Answer from the drawing. Dimensions are ordinates in mm from the lowest x, y and z of the part. Coordinates: 2 decimals unless noted, no trailing zeros. Order: outer loops, then holes, each group sorted by start corner. A loop starts at its lowest first (then second) coordinate and runs counter-clockwise, first axis right, second up. Notation, with made-up numbers: (57, -6) -> (116, -6) arc R27 cw to (116, 23) -> close; hole circle Ø10 at (85.5, -17.5). An arc over 180 degrees is marked (long way). Answer as a JSON object with one key per item and string values. Group by question number.
1) Consider L1, parallel to Z at x = 4, y = 1.2; L2, parallel to Z at x = 26, y = 1; L3, parallel to X at y = 0.4, z = 37. Determine where each line is inside the solid, lowest interval first.
2) Section C-C on z = 67 is taken. Determine the outline of the cut face in (x, y).
3) Section D-D on z = 35.5 is taken. Determine the outline of the cut face in (x, y), and give its area (3 significant figures).
4) Section A-A on y = 1.45 is taken. Determine the outline of the cut face in (x, z).
5) Section B-B on x = 4 is taken. Determine the outline of the cut face in (y, z), and give its area (3 significant figures).
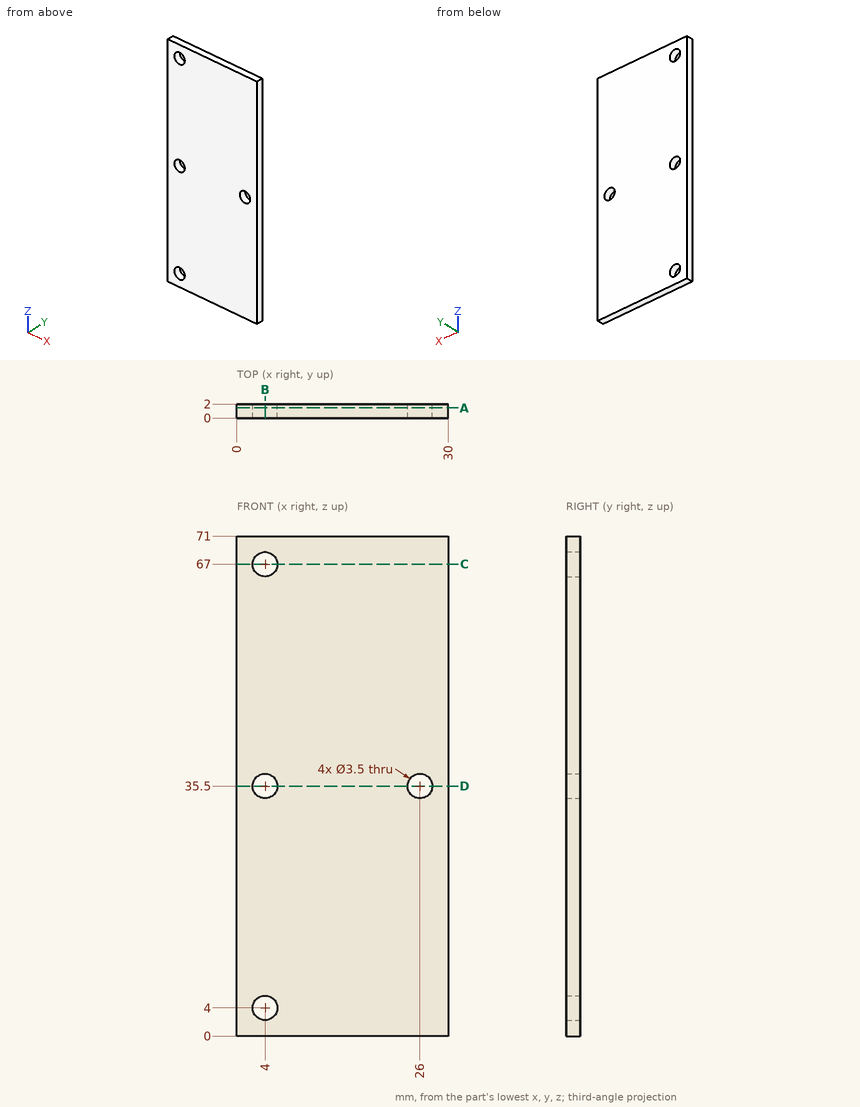
Worked answers:
{
 "1": {"L1": "z = 0 to 2.25, 5.75 to 33.75, 37.25 to 65.25, 68.75 to 71", "L2": "z = 0 to 33.75, 37.25 to 71", "L3": "x = 0 to 3.1, 4.9 to 25.1, 26.9 to 30"},
 "2": {"outline": "(0, 0) -> (2.25, 0) -> (2.25, 2) -> (0, 2) -> close; (5.75, 0) -> (30, 0) -> (30, 2) -> (5.75, 2) -> close"},
 "3": {"outline": "(0, 0) -> (2.25, 0) -> (2.25, 2) -> (0, 2) -> close; (5.75, 0) -> (24.25, 0) -> (24.25, 2) -> (5.75, 2) -> close; (27.75, 0) -> (30, 0) -> (30, 2) -> (27.75, 2) -> close", "area": "46.0 mm²"},
 "4": {"outline": "(0, 0) -> (30, 0) -> (30, 71) -> (0, 71) -> close; hole circle Ø3.5 at (4, 4); hole circle Ø3.5 at (4, 35.5); hole circle Ø3.5 at (4, 67); hole circle Ø3.5 at (26, 35.5)"},
 "5": {"outline": "(0, 0) -> (2, 0) -> (2, 2.25) -> (0, 2.25) -> close; (0, 5.75) -> (2, 5.75) -> (2, 33.75) -> (0, 33.75) -> close; (0, 37.25) -> (2, 37.25) -> (2, 65.25) -> (0, 65.25) -> close; (0, 68.75) -> (2, 68.75) -> (2, 71) -> (0, 71) -> close", "area": "121 mm²"}
}
